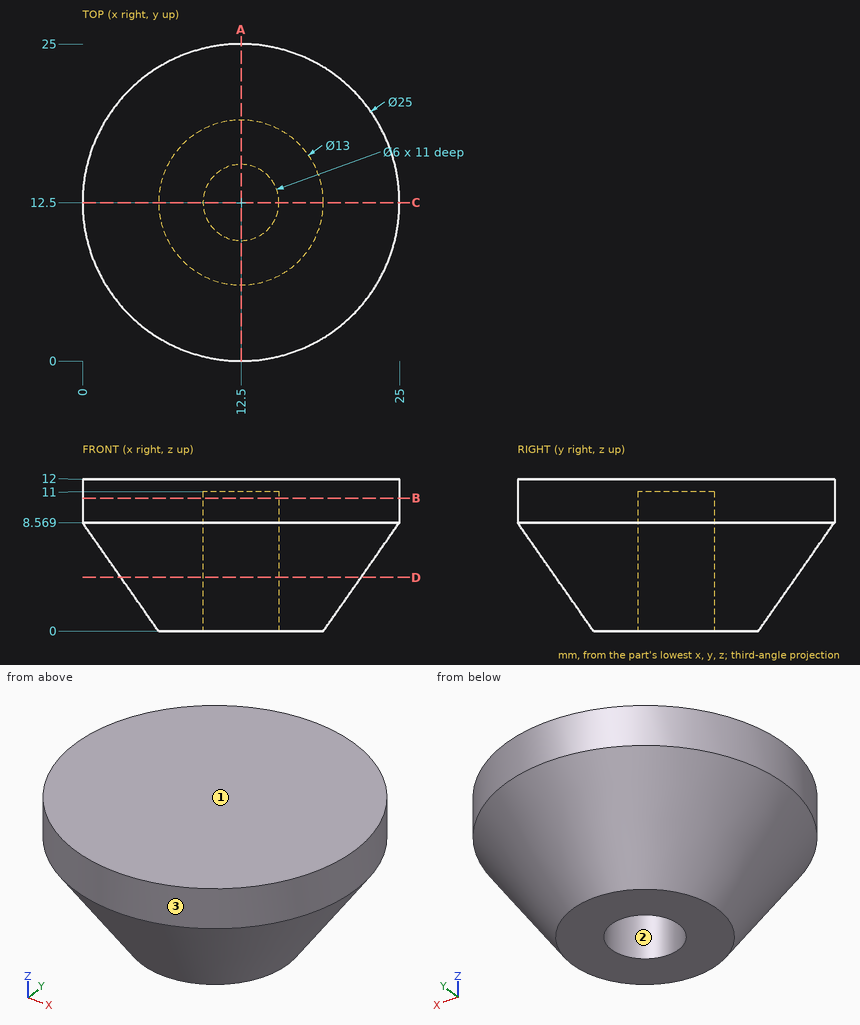
Geometry check sheet. Reference: drawing and pictorial views, mm from the part's lowest x, y, z. Give positions to 0.01 mm unless a question says otherwise; leave off trailing zeros. Write each loop counter-clockwise with the first axis right and the second up, starting at its lowest first coordinate (ties: lowest second). Pieces come first, ordered by that corner, then holes. Notation, with made-up numbers: M 75,-20 L 120,-20 A25 cw 120,-4 Z; hole C 6,-32.75 d7. An arc over 180 degrees is marked long. Put each result on its own line as item: value. Start each with the question number.
1. Section check A-A (x = 12.5). Record the cut outline in (y, z), and give its area (3 significant figures).
2. Go/stop test with flat-tipped pins: pin 1 Ø5 at (x, y) = (19, 10.5) entering from -Z; pin 2 Ø1 at (y, z) = (5.5, 9) entering from +X; pin 3 Ø6 at (x, z) = (17.5, 8) entering from -Y; pin 4 Ø4 at (y, z) = (9.5, 3) entering from +X. Record where each tip stops, or that it passes through.
3. Draft check along X on the marked faces 1, 2 and 3. Enter one of: +X half, -X half, draft (parallel to the pull), parting line (faces both ways), or undercut.
4. Section check D-D (z = 4.25). Record the cut outline in (x, y), and give its area (3 significant figures).
5. Scan lines: line 1 along Y through (x, z) = (10.75, 7); line 2 along X through (y, z) = (10.25, 1.5) (1 decimal); line 3 along Y through (x, z) = (9.75, 6.25). Record each from-to range of solid material in increasing order. Write a range as [from, to].
6. Section check B-B (z = 10.5). Record the cut outline in (x, y), and give its area (3 significant figures).
Answer list:
1. outline: M 0,8.57 L 6,0 L 9.5,0 L 9.5,11 L 15.5,11 L 15.5,0 L 19,0 L 25,8.57 L 25,12 L 0,12 Z
1. area: 183 mm2
2. pin 1: z = 0
2. pin 2: x = 23.18
2. pin 3: y = 0.17
2. pin 4: x = 22.14
3. face 1: draft
3. face 2: undercut
3. face 3: parting line
4. outline: C 12.5,12.5 d18.95; hole C 12.5,12.5 d6
4. area: 254 mm2
5. line 1: [1.23, 10.06], [14.94, 23.77]
5. line 2: [5.3, 10.5], [14.5, 19.7]
5. line 3: [1.98, 11.3], [13.7, 23.02]
6. outline: C 12.5,12.5 d25; hole C 12.5,12.5 d6
6. area: 463 mm2
